Autodesk Fusion 360 part; units mm, degrees
sketch "Sketch1" plane through (0, 0, 0) normal (0, 0, 1) x (1, 0, 0)
  line L0 (1.7898, -44) -> (-40, -44)
  line L1 (-40, 44) -> (1.7898, 44)
  line L2 (-40, 44) -> (-27, 44)
  line L3 (-27, -44) -> (-40, -44)
  line L4 (-27, 22) -> (-24, 22)
  line L5 (-24, -22) -> (-27, -22)
  line L6 (-24, 5) -> (40, 5)
  line L7 (40, 5) -> (40, -5)
  line L8 (40, -5) -> (-24, -5)
  line L9 (-24, 5) -> (-20, 5)
  line L10 (-20, 5) -> (-20, -5)
  line L11 (-20, -5) -> (-24, -5)
  circle A0 centre (-47, 0) radius 9.5
  circle A1 centre (4, 25) radius 5
  circle A2 centre (4, -25) radius 5
  line L12 (49.5, 16.4545) -> (1.7898, 44)
  line L13 (49.5, -16.4545) -> (1.7898, -44)
  arc A3 (-40, 17.6635) -> (-40, -17.6635) centre (-47, 0) ccw
  line L14 (4.5455, -5) -> (4, -4.4) construction
  line L15 (4, -42.7239) -> (4, -44) construction
  line L16 (4, 5) -> (4, 4.4) construction
  line L17 (4, -4.4) -> (4, -5) construction
  line L18 (4, 4.4) -> (4.5455, 5) construction
  line L19 (-56.5, 0) -> (-59, 0) construction
  line L20 (-20, 0) -> (-27, 0) construction
  line L21 (-37.5, 0) -> (-40, 0) construction
  line L22 (-40, 0) -> (-37.5, 0) construction
  line L23 (-27, 0) -> (-24, 0) construction
  line L24 (40, 5) -> (40, -5)
  arc A4 (49.5, -16.4545) -> (49.5, 16.4545) centre (40, 0) ccw
  line L25 (-24, 22) -> (-24, 5)
  line L26 (-24, -5) -> (-24, -22)
  line L27 (-40, -44) -> (-40, -17.6635)
  line L28 (-40, 17.6635) -> (-40, 44)
  line L29 (-40, -44) -> (-40, -17.6635)
  line L30 (-40, 17.6635) -> (-40, 44)
  line L31 (-27, 44) -> (-27, 22)
  line L32 (-27, -22) -> (-27, -44)
  dimension "d2" = 88
  dimension "d3" = 13
  dimension "d4" = 3
  dimension "d5" = 44
  dimension "d6" = 22
  dimension "d7" = 64
  dimension "d8" = 10
  dimension "d9" = 17
  dimension "d10" = 4
  dimension "d12" = 19
  dimension "d13" = 38
  dimension "d17" = 10
  dimension "d18" = 10
extrude "Extrude1" add sketch "Sketch1" along normal blind 10 contours L0 L1 L4 L5 L6 L7 L8 L9 L11 L12 L13 L24 A4 L25 L26 L31 L32
extrude "Extrude2" add sketch "Sketch1" along normal blind 10 contours L6 L7 L8 L10 L24
extrude "Extrude3" add sketch "Sketch1" along normal blind 40 contours L0 L1 L2 L3 L4 L5 L6 L8 L9 L10 L11 A3 L25 L26 L27 L28 L29 L30 L31 L32
fillet "Fillet1" radius 6 1 edges at (-40, -17.6635, 20)
fillet "Fillet2" radius 6 1 edges at (-40, 17.6635, 20)
fillet "Fillet3" radius 3 1 edges at (-27, -22, 25)
fillet "Fillet4" radius 3 1 edges at (-27, 22, 25)
fillet "Fillet5" radius 13 1 edges at (1.7898, 44, 5)
sketch "Sketch2" plane through (0, 0, 0) normal (0, 1, 0) x (1, 0, 0)
  line L0 (39.6527, -10.1952) -> (-20.3473, -10.1952)
  line L1 (-20.3473, -10.1952) -> (-20.3473, -40.1952)
  line L2 (-20.3473, -40.1952) -> (39.6527, -10.1952)
  dimension "d36" = 60
  dimension "d37" = 30
extrude "Extrude4" add sketch "Sketch2" along normal mid plane 10
equation "d5 = 3 mm + 38 mm + 3 mm"
equation "d7 = 67 mm - 3 mm"
equation "d9 = 14 mm + 3 mm"
equation "d36 = 67 mm - 3 mm - 4 mm"
equation "d37 = 40 mm - 10 mm"
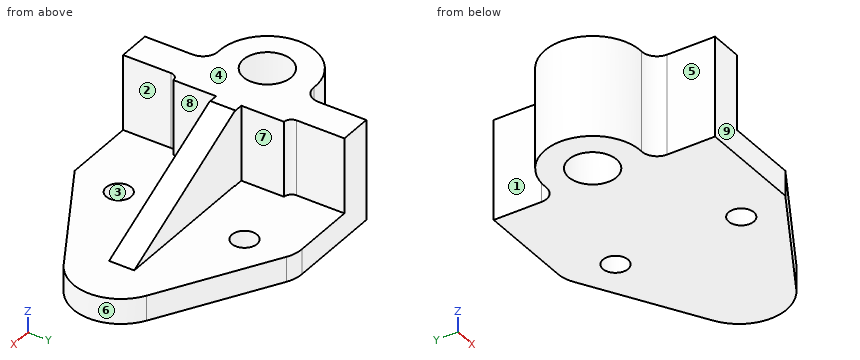
Verification items for the finished model (mm, model axes). Face numbers are marked on the shaded views. A direction names the side the tool comes from. Give positions to 0.01 mm unless a question says otherwise; leave off trailing zeros. Write each loop counter-clockwise with the first axis right and the second up, starting at its lowest first coordinate (ties: lowest second). Pieces come first, ordered by that corner, then holes.
(1) Gauge pin test, flat ends, axial feed: pin 1 (1.5 mm diameter, centred on x = 46, z = 5, fed in from -Y); pin 2 (24.5 mm diameter, centred on x = -47, y = 0, fed in from +Z); pin 3 (21 mm diameter, centred on y = 36, z = 15.5, fed in from -X). Record the tip position at first contact, or that the pin passes through.
(2) Cross-section at A-A (y = 27.5). Enter the section's corners in (x, z).
(3) Cross-section at D-D (z = 4). Enter the section's corners in (x, y), plus the area to 3 significant figures.
(4) Access from +Z, -Z, +X, -X, +Y, -Y to the whole of each face (thin tool, end or side, straight path). Record for the marked faces 5, 6, 7, 8 and 9.
(5) Cross-section at B-B (x = -7.5). Enter the section's corners in (y, z).
(6) Material ranges on line 1 (Y direction, x = 4, z = 6); line 2 (Y direction, x = -47, z = 24); line 3 (X direction, y = -29.5, z = 13), recorded low to high.
(7) Mould release check, pull along X, two halves, no side actions. Record for the marked faces 1, 2, 3 and 4: +X half, -X half, draft (parallel to the pull), parting line (faces both ways), or undercut.
Worked out:
1. pin 1: stops at y = -18.91
1. pin 2: stops at z = 40
1. pin 3: stops at x = -40
2. outline: (-40, 0) - (-0.33, 0) - (-0.33, 10) - (-27, 10) - (-27, 40) - (-40, 40) - close; (8.33, 0) - (30.37, 0) - (30.37, 10) - (8.33, 10) - close
3. outline: (-46.24, -18.98) arc R6 cw to (-40, -24.98) - (-40, -44) - (1.79, -44) - (49.5, -16.45) arc R19 ccw to (49.5, 16.45) - (4.81, 42.26) arc R13 ccw to (-1.69, 44) - (-40, 44) - (-40, 24.98) arc R6 cw to (-46.24, 18.98) arc R19 ccw (long way) to start; hole circle Ø19 at (-47, 0); hole circle Ø10 at (4, -25); hole circle Ø10 at (4, 25)
3. area: 7,190 mm2
4. face 5: +Z, -Z, -X, -Y
4. face 6: +Z, -Z, +X
4. face 7: +Z, +X, +Y
4. face 8: +Z, +X, -Y
4. face 9: +Z, -Z, +X, -X, -Y
5. outline: (-44, 0) - (44, 0) - (44, 10) - (-44, 10) - close; (-5, 10.2) - (5, 10.2) - (5, 33.77) - (-5, 33.77) - close
6. line 1: y = -42.72 to -30, -20 to 20, 30 to 42.69
6. line 2: y = -19 to -9.5, 9.5 to 19
6. line 3: x = -40 to -27
7. face 1: -X half
7. face 2: +X half
7. face 3: undercut
7. face 4: draft
